Geometry check sheet. Reference: the model listing, model coordinates, mm. Give positions to 0.01 mm unless a question says otherwise; leave off trailing zeros. Loops run counter-clockwise (first coordinate to the right, second up) from the corner with the lowest first, then second, coordinate; pieces in that order, holes last. Notation, with made-up numbers: (-27, -4.75) - (23, -4.75) arc R23 cw to (23, 27.25) - close; hole circle Ø3 at (60.5, -20). An arc over 180 degrees is marked (long way). Use a Markdown table: item, result. Add a question column.
1. Material ranges on L1, parallel to Y at x = -89.5, z = -47; L2, parallel to Z at x = -827, y = -825; L3, parallel to X at y = -740.5, z = -70.5, recorded low to high.
2. Cross-section at A-A on z = -35. Enter the section's corners in (x, y).
3. Depth check by flat-ended pin: P1, Ø12, axis at y = -748, z = -75, coming from the +X side; P2, Ø1, axis at x = -435, y = -957, coming from the -Z side; P3, Ø13, axis at y = -673, z = 79, coming from the +X side. Enter the tip coordinate at first touch or a pass-through.
4. Cross-section at B-B on y = -706. Enter the section's corners in (x, z), and give its area (3 significant figures).
5. Cross-section at C-C on x = -395.5. Enter the section's corners in (y, z), and give its area (3 significant figures).
6. Cross-section at D-D on y = -1239. Enter the section's corners in (x, z).
from build123d import *

# Parameters (mm, degrees)
BOSS_EXTRUDE2_DEPTH = 57.15
BOSS_EXTRUDE3_DEPTH = 44
CUT_EXTRUDE1_DEPTH  = 44
FILLET1_R           = 10
BOSS_EXTRUDE4_DEPTH = 100
SKETCH8_W           = 58.558244651631945
SKETCH8_H           = 158.82756414249673
CUT_EXTRUDE3_DEPTH  = 70


with BuildPart() as part:
    # Sketch1 → Boss-Extrude2 (new body)
    with BuildSketch(Plane.XY):
        Polygon((0, 0), (0, 446.2018372120283), (-1100, 446.2018372120282), (-1100, -1585.7981627879717), (0, -1585.7981627879717), align=None)
    extrude(amount=BOSS_EXTRUDE2_DEPTH)

    # Sketch4 → Boss-Extrude3 (add)
    with BuildSketch(Plane.XY.offset(57.15)):
        Polygon((-79.99999999999993, -603.7981627879718), (-49.999999999999936, -603.7981627879718), (-49.999999999999915, -785.7981627879718), (-79.9999999999999, -785.7981627879718), align=None)
    extrude(amount=BOSS_EXTRUDE3_DEPTH)

    # Sketch5 → Cut-Extrude1 (cut)
    with BuildSketch(Plane.ZY.offset(80.00000000000003)):
        Polygon((83.14999999999999, -624.7981627879717), (57.150000000000006, -624.7981627879717), (57.15, -764.7981627879717), (83.15, -764.7981627879717), align=None)
    extrude(amount=-CUT_EXTRUDE1_DEPTH, mode=Mode.SUBTRACT)

    # Fillet1
    # the kernel refuses this fillet: 10 mm, written as the material it takes off along each edge
    with BuildSketch(Plane(origin=(-69.99999999999993, -613.7981627879718, 91.15), x_dir=(-1, -1.6e-16, 0), z_dir=(0, 1, 0))) as fillet1_piece_1_section:
        Polygon((0, 0), (FILLET1_R, 0), (FILLET1_R, FILLET1_R), (0, FILLET1_R), align=None)
    fillet1_piece_1 = extrude(amount=FILLET1_R, mode=Mode.PRIVATE)
    fillet1_piece_1 = fillet1_piece_1 - Plane(origin=(-69.99999999999993, -613.7981627879718, 91.15), x_dir=(0.7071067811865475, 0, -0.7071067811865475), z_dir=(0, 1, 0)) * Sphere(FILLET1_R, mode=Mode.PRIVATE)
    add(fillet1_piece_1, mode=Mode.SUBTRACT)
    with BuildSketch(Plane(origin=(-69.9999999999999, -775.7981627879718, 91.15), x_dir=(0, 0, 1), z_dir=(-1, -1.6e-16, 0))) as fillet1_piece_2_section:
        Polygon((0, 0), (FILLET1_R, 0), (FILLET1_R, -FILLET1_R), (0, -FILLET1_R), align=None)
    fillet1_piece_2 = extrude(amount=FILLET1_R, mode=Mode.PRIVATE)
    fillet1_piece_2 = fillet1_piece_2 - Plane(origin=(-69.9999999999999, -775.7981627879718, 91.15), x_dir=(0, 0.7071067811865475, -0.7071067811865475), z_dir=(-1, -1.6e-16, 0)) * Sphere(FILLET1_R, mode=Mode.PRIVATE)
    add(fillet1_piece_2, mode=Mode.SUBTRACT)
    with BuildSketch(Plane(origin=(-49.999999999999915, -785.7981627879718, 57.15), x_dir=(-1, 0, 0), z_dir=(0, 0, 1))) as fillet1_piece_3:
        with BuildLine():
            CenterArc((FILLET1_R, -FILLET1_R), FILLET1_R, 90, 90)
            Line((0, -FILLET1_R), (0, 0))
            Line((0, 0), (FILLET1_R, 0))
        make_face()
    extrude(amount=69, mode=Mode.SUBTRACT)
    with BuildSketch(Plane(origin=(-49.999999999999936, -603.7981627879718, 57.15), x_dir=(0, -1, 0), z_dir=(0, 0, 1))) as fillet1_piece_4:
        with BuildLine():
            CenterArc((FILLET1_R, -FILLET1_R), FILLET1_R, 90, 90)
            Line((0, -FILLET1_R), (0, 0))
            Line((0, 0), (FILLET1_R, 0))
        make_face()
    extrude(amount=69, mode=Mode.SUBTRACT)
    with BuildSketch(Plane(origin=(-79.99999999999993, -603.7981627879718, 57.15), x_dir=(1, 0, 0), z_dir=(0, 0, 1))) as fillet1_piece_5:
        with BuildLine():
            CenterArc((FILLET1_R, -FILLET1_R), FILLET1_R, 90, 90)
            Line((0, -FILLET1_R), (0, 0))
            Line((0, 0), (FILLET1_R, 0))
        make_face()
    extrude(amount=34.00000000000001, mode=Mode.SUBTRACT)
    with BuildSketch(Plane(origin=(-79.9999999999999, -785.7981627879718, 57.15), x_dir=(1, 0, 0), z_dir=(0, 0, 1))) as fillet1_piece_6:
        with BuildLine():
            CenterArc((FILLET1_R, FILLET1_R), FILLET1_R, 180, 90)
            Line((0, FILLET1_R), (0, 0))
            Line((0, 0), (FILLET1_R, 0))
        make_face()
    extrude(amount=34.00000000000001, mode=Mode.SUBTRACT)
    with BuildSketch(Plane(origin=(-69.99999999999993, -603.7981627879718, 101.15), x_dir=(0, 0, -1), z_dir=(1, 0, 0))) as fillet1_piece_7:
        with BuildLine():
            CenterArc((FILLET1_R, -FILLET1_R), FILLET1_R, 90, 90)
            Line((0, -FILLET1_R), (0, 0))
            Line((0, 0), (FILLET1_R, 0))
        make_face()
    extrude(amount=44.99999999999999, mode=Mode.SUBTRACT)
    with BuildSketch(Plane(origin=(-79.9999999999999, -775.7981627879718, 101.15), x_dir=(0, 0, -1), z_dir=(-1.6e-16, 1, 0))) as fillet1_piece_8:
        with BuildLine():
            CenterArc((FILLET1_R, -FILLET1_R), FILLET1_R, 90, 90)
            Line((0, -FILLET1_R), (0, 0))
            Line((0, 0), (FILLET1_R, 0))
        make_face()
    extrude(amount=162, mode=Mode.SUBTRACT)
    with BuildSketch(Plane(origin=(-24.999999999999915, -785.7981627879718, 101.15), x_dir=(0, 0, -1), z_dir=(-1, 0, 0))) as fillet1_piece_9:
        with BuildLine():
            CenterArc((FILLET1_R, -FILLET1_R), FILLET1_R, 90, 90)
            Line((0, -FILLET1_R), (0, 0))
            Line((0, 0), (FILLET1_R, 0))
        make_face()
    extrude(amount=44.999999999999986, mode=Mode.SUBTRACT)
    with BuildSketch(Plane(origin=(-79.99999999999991, -764.7981627879717, 57.15000000000002), x_dir=(1.42e-15, -1, 0), z_dir=(0, 0, 1))) as fillet1_piece_10:
        with BuildLine():
            CenterArc((FILLET1_R, FILLET1_R), FILLET1_R, 180, 89.99999999999989)
            Line((1.421e-14, FILLET1_R), (0, 0))
            Line((0, 0), (FILLET1_R, 0))
        make_face()
    extrude(amount=25.999999999999986, mode=Mode.SUBTRACT)
    with BuildSketch(Plane(origin=(-79.99999999999993, -624.7981627879717, 83.14999999999999), x_dir=(0, 1, 0), z_dir=(0, 0, -1))) as fillet1_piece_11:
        with BuildLine():
            CenterArc((FILLET1_R, FILLET1_R), FILLET1_R, 180, 90)
            Line((0, FILLET1_R), (0, 0))
            Line((0, 0), (FILLET1_R, 0))
        make_face()
    extrude(amount=25.999999999999986, mode=Mode.SUBTRACT)
    with BuildSketch(Plane(origin=(-79.99999999999991, -764.7981627879717, 83.15), x_dir=(1.42e-15, 1e-16, 1), z_dir=(-1.5e-16, 1, -1e-16))) as fillet1_piece_12:
        with BuildLine():
            CenterArc((FILLET1_R, FILLET1_R), FILLET1_R, 180, 89.99999999999989)
            Line((1.421e-14, FILLET1_R), (0, 0))
            Line((0, 0), (FILLET1_R, 0))
        make_face()
    extrude(amount=140, mode=Mode.SUBTRACT)
    with BuildSketch(Plane(origin=(-49.999999999999915, -764.7981627879717, 83.15), x_dir=(0, -1, 0), z_dir=(0, 0, -1))) as fillet1_piece_13:
        with BuildLine():
            CenterArc((FILLET1_R, FILLET1_R), FILLET1_R, 180, 90)
            Line((0, FILLET1_R), (0, 0))
            Line((0, 0), (FILLET1_R, 0))
        make_face()
    extrude(amount=26, mode=Mode.SUBTRACT)
    with BuildSketch(Plane(origin=(-49.999999999999936, -624.7981627879717, 57.150000000000006), x_dir=(0, 1, 0), z_dir=(0, 0, 1))) as fillet1_piece_14:
        with BuildLine():
            CenterArc((FILLET1_R, FILLET1_R), FILLET1_R, 180.00000000000003, 90)
            Line((0, FILLET1_R), (0, 0))
            Line((0, 0), (FILLET1_R, 0))
        make_face()
    extrude(amount=25.999999999999986, mode=Mode.SUBTRACT)
    with BuildSketch(Plane(origin=(-49.999999999999936, -624.7981627879717, 83.15), x_dir=(0, 1e-16, 1), z_dir=(1.2e-16, -1, 1e-16))) as fillet1_piece_15:
        with BuildLine():
            CenterArc((FILLET1_R, FILLET1_R), FILLET1_R, 180, 90)
            Line((0, FILLET1_R), (0, 0))
            Line((0, 0), (FILLET1_R, 0))
        make_face()
    extrude(amount=140, mode=Mode.SUBTRACT)
    with BuildSketch(Plane(origin=(-79.99999999999991, -764.7981627879717, 57.15000000000002), x_dir=(1.42e-15, -1, 0), z_dir=(0, 0, 1))) as fillet1_piece_16a_section:
        with BuildLine():
            CenterArc((FILLET1_R, FILLET1_R), FILLET1_R, 180, 89.99999999999989)
            Line((1.421e-14, FILLET1_R), (0, 0))
            Line((0, 0), (FILLET1_R, 0))
        make_face()
    fillet1_piece_16a = extrude(amount=50.999999999999986, mode=Mode.PRIVATE)
    fillet1_piece_16a = split(fillet1_piece_16a, bisect_by=Plane(origin=(-77.7360488573316, -767.0621139306398, 83.15), z_dir=(0, 1e-16, 1)), keep=Keep.TOP, mode=Mode.PRIVATE)
    with BuildSketch(Plane(origin=(-79.9999999999999, -789.7981627879717, 83.15), x_dir=(0, 1e-16, 1), z_dir=(-1.5e-16, 1, -1e-16))) as fillet1_piece_16b_section:
        with BuildLine():
            CenterArc((FILLET1_R, FILLET1_R), FILLET1_R, 180, 90)
            Line((0, FILLET1_R), (0, 0))
            Line((0, 0), (FILLET1_R, 0))
        make_face()
    fillet1_piece_16b = extrude(amount=165, mode=Mode.PRIVATE)
    fillet1_piece_16b = split(fillet1_piece_16b, bisect_by=Plane(origin=(-77.73604885733165, -764.7981627879717, 85.41395114266827), z_dir=(1.5e-16, -1, 0)), keep=Keep.TOP, mode=Mode.PRIVATE)
    fillet1_piece_16 = fillet1_piece_16a & fillet1_piece_16b
    add(fillet1_piece_16, mode=Mode.SUBTRACT)
    with BuildSketch(Plane(origin=(-79.99999999999991, -764.7981627879717, 83.15), x_dir=(1.42e-15, 1e-16, 1), z_dir=(-1.5e-16, 1, -1e-16))) as fillet1_piece_17a_section:
        with BuildLine():
            CenterArc((FILLET1_R, FILLET1_R), FILLET1_R, 180, 89.99999999999989)
            Line((1.421e-14, FILLET1_R), (0, 0))
            Line((0, 0), (FILLET1_R, 0))
        make_face()
    fillet1_piece_17a = extrude(amount=165, mode=Mode.PRIVATE)
    fillet1_piece_17a = split(fillet1_piece_17a, bisect_by=Plane(origin=(-77.73604885733167, -624.7981627879717, 85.41395114266825), z_dir=(-1.5e-16, 1, 0)), keep=Keep.TOP, mode=Mode.PRIVATE)
    with BuildSketch(Plane(origin=(-79.99999999999993, -624.7981627879717, 108.14999999999998), x_dir=(0, 1, 0), z_dir=(0, 0, -1))) as fillet1_piece_17b_section:
        with BuildLine():
            CenterArc((FILLET1_R, FILLET1_R), FILLET1_R, 180, 90)
            Line((0, FILLET1_R), (0, 0))
            Line((0, 0), (FILLET1_R, 0))
        make_face()
    fillet1_piece_17b = extrude(amount=50.999999999999986, mode=Mode.PRIVATE)
    fillet1_piece_17b = split(fillet1_piece_17b, bisect_by=Plane(origin=(-77.73604885733164, -622.5342116453035, 83.14999999999999), z_dir=(0, 1e-16, 1)), keep=Keep.TOP, mode=Mode.PRIVATE)
    fillet1_piece_17 = fillet1_piece_17a & fillet1_piece_17b
    add(fillet1_piece_17, mode=Mode.SUBTRACT)
    with BuildSketch(Plane(origin=(-49.999999999999936, -624.7981627879717, 83.15), x_dir=(0, 1e-16, 1), z_dir=(1.2e-16, -1, 1e-16))) as fillet1_piece_18a_section:
        with BuildLine():
            CenterArc((FILLET1_R, FILLET1_R), FILLET1_R, 180, 90)
            Line((0, FILLET1_R), (0, 0))
            Line((0, 0), (FILLET1_R, 0))
        make_face()
    fillet1_piece_18a = extrude(amount=165, mode=Mode.PRIVATE)
    fillet1_piece_18a = split(fillet1_piece_18a, bisect_by=Plane(origin=(-52.26395114266817, -764.7981627879717, 85.41395114266827), z_dir=(1.5e-16, -1, 0)), keep=Keep.TOP, mode=Mode.PRIVATE)
    with BuildSketch(Plane(origin=(-49.999999999999915, -764.7981627879717, 108.15), x_dir=(0, -1, 0), z_dir=(0, 0, -1))) as fillet1_piece_18b_section:
        with BuildLine():
            CenterArc((FILLET1_R, FILLET1_R), FILLET1_R, 180, 90)
            Line((0, FILLET1_R), (0, 0))
            Line((0, 0), (FILLET1_R, 0))
        make_face()
    fillet1_piece_18b = extrude(amount=51, mode=Mode.PRIVATE)
    fillet1_piece_18b = split(fillet1_piece_18b, bisect_by=Plane(origin=(-52.2639511426682, -767.0621139306397, 83.15), z_dir=(0, 1e-16, 1)), keep=Keep.TOP, mode=Mode.PRIVATE)
    fillet1_piece_18 = fillet1_piece_18a & fillet1_piece_18b
    add(fillet1_piece_18, mode=Mode.SUBTRACT)
    with BuildSketch(Plane(origin=(-49.999999999999936, -624.7981627879717, 57.150000000000006), x_dir=(0, 1, 0), z_dir=(0, 0, 1))) as fillet1_piece_19a_section:
        with BuildLine():
            CenterArc((FILLET1_R, FILLET1_R), FILLET1_R, 180.00000000000003, 90)
            Line((0, FILLET1_R), (0, 0))
            Line((0, 0), (FILLET1_R, 0))
        make_face()
    fillet1_piece_19a = extrude(amount=50.999999999999986, mode=Mode.PRIVATE)
    fillet1_piece_19a = split(fillet1_piece_19a, bisect_by=Plane(origin=(-52.26395114266823, -622.5342116453035, 83.14999999999999), z_dir=(0, 1e-16, 1)), keep=Keep.TOP, mode=Mode.PRIVATE)
    with BuildSketch(Plane(origin=(-49.999999999999936, -599.7981627879717, 83.14999999999999), x_dir=(0, 1e-16, 1), z_dir=(1.2e-16, -1, 1e-16))) as fillet1_piece_19b_section:
        with BuildLine():
            CenterArc((FILLET1_R, FILLET1_R), FILLET1_R, 179.99999999999997, 90)
            Line((0, FILLET1_R), (0, 0))
            Line((0, 0), (FILLET1_R, 0))
        make_face()
    fillet1_piece_19b = extrude(amount=165, mode=Mode.PRIVATE)
    fillet1_piece_19b = split(fillet1_piece_19b, bisect_by=Plane(origin=(-52.26395114266818, -624.7981627879717, 85.41395114266824), z_dir=(-1.5e-16, 1, 0)), keep=Keep.TOP, mode=Mode.PRIVATE)
    fillet1_piece_19 = fillet1_piece_19a & fillet1_piece_19b
    add(fillet1_piece_19, mode=Mode.SUBTRACT)

    # Sketch6 → Boss-Extrude4 (add)
    with BuildSketch(Plane(origin=(0, 0, 0), x_dir=(-1, 0, 0), z_dir=(0, 0, -1))):
        Polygon((64.99999999999997, -612.0487005102074), (134.99999999999994, -612.0487005102074), (135, -812.0487005102073), (65, -812.0487005102073), align=None)
    extrude(amount=BOSS_EXTRUDE4_DEPTH)

    # Sketch8 → Cut-Extrude3 (cut)
    with BuildSketch(Plane(origin=(-64.99999999999989, 9.02e-15, 0), x_dir=(0, 0, -1), z_dir=(1, -1.4e-16, 0))):
        with Locations((29.279122325815973, -707.3493580183326)):
            Rectangle(SKETCH8_W, SKETCH8_H)
    extrude(amount=-CUT_EXTRUDE3_DEPTH, mode=Mode.SUBTRACT)


solid = part.part
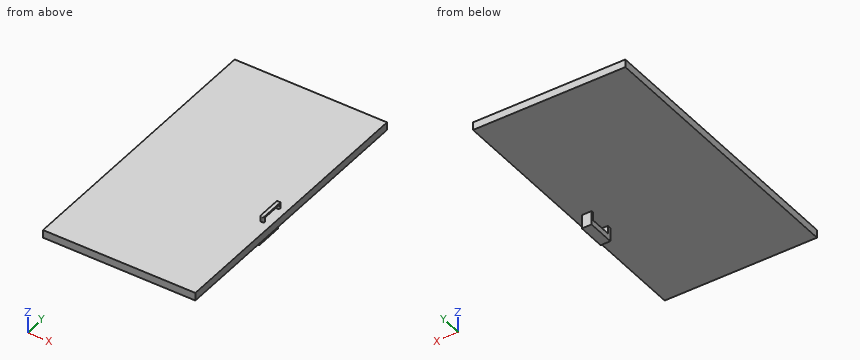
Values found:
| question | item | result |
|---|---|---|
| 1 | L1 | y = -812.05 to -786.76, -627.94 to -612.05 |
| 1 | L2 | z = 0 to 57.15 |
| 1 | L3 | x = -135 to -65 |
| 2 | outline | (-135, -812.05) - (-65, -812.05) - (-65, -786.76) - (-135, -786.76) - close; (-135, -627.94) - (-65, -627.94) - (-65, -612.05) - (-135, -612.05) - close |
| 3 | P1 | stops at x = -65 |
| 3 | P2 | stops at z = 0 |
| 3 | P3 | stops at x = -53.56 |
| 4 | outline | (-1100, 0) - (0, 0) - (0, 57.15) - (-1100, 57.15) - close; (-135, -100) - (-65, -100) - (-65, -58.56) - (-135, -58.56) - close; (-79.95, 92.15) arc R10 ccw to (-70, 83.15) - (-60, 83.15) arc R10 ccw to (-50, 93.15) - (-50, 101.15) - (-70, 101.15) arc R10 ccw to start |
| 4 | area | 66,200 mm2 |
| 5 | outline | (-1585.8, 0) - (446.2, 0) - (446.2, 57.15) - (-1585.8, 57.15) - close |
| 5 | area | 116,000 mm2 |
| 6 | outline | (-1100, 0) - (0, 0) - (0, 57.15) - (-1100, 57.15) - close |
